The listing builds one solid part. Answer for the finished solid, in the listing's coordinates (mm). A direction names the side the tool comes from. Give positions to 0.01 mm unless a question says otherwise; leave off trailing zeros. Order: outer loops, then holes, each group sorted by start corner. A loop starts at its lowest first (then second) coordinate and runs counter-clockwise, first axis right, second up. Notation, with made-up numbers: (37, 85) - (77, 85) arc R25 ccw to (77, 109) - close; hole circle Ø6 at (-25.75, -34.75). An arc over 180 degrees is marked (long way). Answer as CSV lines item,"result". Start each with the question number.
1. Which of the six approach directions +Z, -Z, +X, -X, +Y, -Y give full straight-line access (tool end or side, diameter ignored) to faces 1 (the cylindrical face through (-1.729, -1.502, -4.396)), 2 (the flat face through (0, -4.5, 0)), 3 (the flat face through (-2, -1.2, -3))?
2. Section A-A on z = -7 is taken. Give the vertices of the cut face in (x, y) (3 decimals).
3. Flat-ended cylindrical pins translate along their axes: pin 1 (5 mm diameter, centred on y = -0.5, z = -6, fed in from -X) (3 decimals); pin 2 (1.7 mm diameter, centred on x = 1.75, y = 0, fed in from +Z); pin 3 (2 mm diameter, centred on x = -2, z = -5, fed in from +Y). Find the tip coordinate at first contact, or state that the pin passes through.
4. Consider line 1 along Y through (x, z) = (0.5, 0.5); line 2 along X through (y, z) = (-0.5, -3.75) (3 decimals); line 3 along Y through (x, z) = (-1.75, -7.2). Determine where each line is inside the solid, lowest interval first. Write a range as [from, to].
5. Section C-C on z = -2.25 is taken. Give the vertices of the cut face in (x, y) (3 decimals).
6. Section D-D on y = 0 is taken. Count the separate pieces of the cut face and the enclosed holes in it, and give its area (3 significant figures).
7. Determine the mould class of faces 4 (the flat face through (1.8, 1.3, -7.65)), 5 (the flat face through (-2.65, 0, -2)), 6 (the flat face through (3.5, -0.1, -0.7)) for opening direction X: +X half, -X half, draft (parallel to the pull), parting line (faces both ways), or undercut.
from build123d import *

# Parameters (mm, degrees)
SKETCH_1_W                     = 3.125
SKETCH_1_H                     = 10.4
EXTRUDE_1_DEPTH                = 2.1
CUT_EXTRUDE_1_REACH            = 8.249
SKETCH_2_W                     = 6.25
SKETCH_2_H                     = 9
SKETCH_3_W                     = 1.55
SKETCH_3_H                     = 0.7
CUT_EXTRUDE_2_DEPTH            = 1.05
SKETCH_5_W                     = 1.55
SKETCH_5_H                     = 0.7
CUT_EXTRUDE_4_DEPTH            = 1.05
EXTRUDE_3_DEPTH                = 6.6
SKETCH_9_W                     = 2.8
SKETCH_9_H                     = 7.7
EXTRUDE_4_DEPTH                = 1.3
CUT_EXTRUDE_6_REACH            = 11.424
SKETCH_11_W                    = 1.8
SKETCH_11_H                    = 6.7
CUT_EXTRUDE_9_REACH            = 11.047
SKETCH_14_W                    = 1.8
SKETCH_14_H                    = 2.4
CUT_EXTRUDE_11_REACH           = 14.749
SKETCH_16_W                    = 1.55
SKETCH_16_H                    = 0.6
CUT_EXTRUDE_12_REACH           = 14.749
SKETCH_17_W                    = 1.55
SKETCH_17_H                    = 0.6
EXTRUDE_6_DEPTH                = 0.375
SKETCH_21_W                    = 0.8
SKETCH_21_H                    = 2.5
EXTRUDE_8_DEPTH                = 1.3
HOLE_WIZARD_2_1_2_1_2_D        = 2.1
HOLE_WIZARD_2_1_2_1_2_DEPTH    = 1.2
HOLE_WIZARD_1_5_1_5_1_D        = 1.5
HOLE_WIZARD_1_5_1_5_1_DEPTH    = 2.000025
FILLET_1_R                     = 0.3
PATTERN_LINEAR_1_COUNT         = 2
PATTERN_LINEAR_1_PITCH         = 3.5
FILLET_1_OF_PATTERN_LINEAR_1_R = 0.3


with BuildPart() as part:
    # Эскиз1 → Бобышка-Вытянуть1 (new body)
    with BuildSketch(Plane.XY.offset(1.05)):
        with Locations((-1.5625, 0)):
            Rectangle(SKETCH_1_W, SKETCH_1_H)
    extrude_1 = extrude(amount=-EXTRUDE_1_DEPTH)

    # Эскиз2 → Вырез-Вытянуть1 (cut, up to next)
    with BuildSketch(Plane(origin=(0, 0, -0.45), x_dir=(-1, 0, 0), z_dir=(0, 0, -1)), mode=Mode.PRIVATE) as cut_extrude_1_sk1:
        Rectangle(SKETCH_2_W, SKETCH_2_H)
    cut_extrude_1_tool1 = extrude(cut_extrude_1_sk1.sketch, amount=-CUT_EXTRUDE_1_REACH, mode=Mode.PRIVATE) & part.part
    cut_extrude_1 = cut_extrude_1_tool1.solids().sort_by_distance((0, 0, -0.45))[0]
    add(cut_extrude_1, mode=Mode.SUBTRACT)

    # Эскиз3 → Вырез-Вытянуть2 (cut)
    with BuildSketch(Plane(origin=(0, 0, -0.45), x_dir=(-1, 0, 0), z_dir=(0, 0, -1))):
        with Locations((1.75, 4.85)):
            Rectangle(SKETCH_3_W, SKETCH_3_H)
    cut_extrude_2 = extrude(amount=-CUT_EXTRUDE_2_DEPTH, mode=Mode.SUBTRACT)

    # Эскиз5 → Вырез-Вытянуть4 (cut)
    with BuildSketch(Plane(origin=(0, 0, -0.45), x_dir=(-1, 0, 0), z_dir=(0, 0, -1))):
        with Locations((1.75, -4.85)):
            Rectangle(SKETCH_5_W, SKETCH_5_H)
    cut_extrude_4 = extrude(amount=-CUT_EXTRUDE_4_DEPTH, mode=Mode.SUBTRACT)

    # Эскиз8 → Бобышка-Вытянуть3 (add)
    with BuildSketch(Plane(origin=(0, 0, -7.65), x_dir=(-1, 0, 0), z_dir=(0, 0, -1))):
        with BuildLine():
            Line((3.125, 2.05), (0.375, 2.05))
            Line((0.375, 2.05), (0.375, -2.05))
            ThreePointArc((0.375, -2.05), (1.75, -1.502368755), (3.125, -2.05))
            Line((3.125, -2.05), (3.125, 2.05))
        make_face()
    extrude_3 = extrude(amount=-EXTRUDE_3_DEPTH)

    # Эскиз9 → Бобышка-Вытянуть4 (add)
    with BuildSketch(Plane.XY.offset(0.85)):
        with Locations((-1.75, 0)):
            Rectangle(SKETCH_9_W, SKETCH_9_H)
    extrude_4 = extrude(amount=-EXTRUDE_4_DEPTH)

    # Эскиз11 → Вырез-Вытянуть6 (cut, up to next)
    with BuildSketch(Plane(origin=(0, 0, -0.45), x_dir=(-1, 0, 0), z_dir=(0, 0, -1)), mode=Mode.PRIVATE) as cut_extrude_6_sk1:
        with Locations((1.75, 0)):
            Rectangle(SKETCH_11_W, SKETCH_11_H)
    cut_extrude_6_tool1 = extrude(cut_extrude_6_sk1.sketch, amount=-CUT_EXTRUDE_6_REACH, mode=Mode.PRIVATE) & part.part
    cut_extrude_6 = cut_extrude_6_tool1.solids().sort_by_distance((-1.75, 0, -0.45))[0]
    add(cut_extrude_6, mode=Mode.SUBTRACT)

    # Эскиз14 → Вырез-Вытянуть9 (cut, up to next)
    with BuildSketch(Plane(origin=(0, 0, -5.65), x_dir=(-1, 0, 0), z_dir=(0, 0, -1)), mode=Mode.PRIVATE) as cut_extrude_9_sk1:
        with Locations((1.75, 0)):
            Rectangle(SKETCH_14_W, SKETCH_14_H)
    cut_extrude_9_tool1 = extrude(cut_extrude_9_sk1.sketch, amount=-CUT_EXTRUDE_9_REACH, mode=Mode.PRIVATE) & part.part
    cut_extrude_9 = cut_extrude_9_tool1.solids().sort_by_distance((-1.75, 0, -5.65))[0]
    add(cut_extrude_9, mode=Mode.SUBTRACT)

    # Эскиз16 → Вырез-Вытянуть11 (cut, up to next)
    with BuildSketch(Plane(origin=(0, -4.5, 0), x_dir=(1, 0, 0), z_dir=(0, 1, 0)), mode=Mode.PRIVATE) as cut_extrude_11_sk1:
        with Locations((-1.75, 0.75)):
            Rectangle(SKETCH_16_W, SKETCH_16_H)
    cut_extrude_11_tool1 = extrude(cut_extrude_11_sk1.sketch, amount=-CUT_EXTRUDE_11_REACH, mode=Mode.PRIVATE) & part.part
    cut_extrude_11 = cut_extrude_11_tool1.solids().sort_by_distance((-1.75, -4.5, -0.75))[0]
    add(cut_extrude_11, mode=Mode.SUBTRACT)

    # Эскиз17 → Вырез-Вытянуть12 (cut, up to next)
    with BuildSketch(Plane.XZ.offset(-4.5), mode=Mode.PRIVATE) as cut_extrude_12_sk1:
        with Locations((-1.75, -0.75)):
            Rectangle(SKETCH_17_W, SKETCH_17_H)
    cut_extrude_12_tool1 = extrude(cut_extrude_12_sk1.sketch, amount=-CUT_EXTRUDE_12_REACH, mode=Mode.PRIVATE) & part.part
    cut_extrude_12 = cut_extrude_12_tool1.solids().sort_by_distance((-1.75, 4.5, -0.75))[0]
    add(cut_extrude_12, mode=Mode.SUBTRACT)

    # Эскиз19 → Бобышка-Вытянуть6 (add)
    with BuildSketch(Plane(origin=(-3.5, 0, 0), x_dir=(0, -1, 0), z_dir=(-1, 0, 0))):
        Polygon((1.65, -1.046361901), (5.2, -1.046361901), (5.2, 1.05), (4.5, 1.05), (4.5, -0.45), (-4.5, -0.45), (-4.5, 1.05), (-5.2, 1.05), (-5.2, -1.046361901), align=None)
    extrude_6 = extrude(amount=-EXTRUDE_6_DEPTH)

    # Эскиз21 → Бобышка-Вытянуть8 (add)
    with BuildSketch(Plane(origin=(0, 3.35, 0), x_dir=(1, 0, 0), z_dir=(0, 1, 0))):
        with Locations((-1.75, 6.4)):
            Rectangle(SKETCH_21_W, SKETCH_21_H)
    extrude_8 = extrude(amount=-EXTRUDE_8_DEPTH)

    # Диаметр отверстия Ø2.1 (2.1)2
    with Locations(Plane(origin=(0, 0, -7.65), x_dir=(-1, 0, 0), z_dir=(0, 0, -1))):
        with Locations((1.75, 0)):
            hole_wizard_2_1_2_1_2 = Hole(HOLE_WIZARD_2_1_2_1_2_D / 2, depth=HOLE_WIZARD_2_1_2_1_2_DEPTH)

    # Диаметр отверстия Ø1.5 (1.5)1
    with Locations(Plane.XY.offset(-5.65)):
        with Locations((-1.75, 0)):
            hole_wizard_1_5_1_5_1 = Hole(HOLE_WIZARD_1_5_1_5_1_D / 2, depth=HOLE_WIZARD_1_5_1_5_1_DEPTH)

    # Скругление1
    fillet_1_edges = [part.edges().sort_by_distance(p)[0] for p in [
        (-2.8, 0, -6.45),
    ]]
    fillet(fillet_1_edges, radius=FILLET_1_R - 0.0001)  # a hair under: the kernel refuses the full size

    # Линейный массив1: Бобышка-Вытянуть1, Вырез-Вытянуть1, Вырез-Вытянуть2, Вырез-Вытянуть4, Бобышка-Вытянуть3, Бобышка-Вытянуть4, Вырез-Вытянуть6, Вырез-Вытянуть9, Вырез-Вытянуть11, Вырез-Вытянуть12, Бобышка-Вытянуть6, Бобышка-Вытянуть8, Диаметр отверстия Ø2.1 (2.1)2, Диаметр отверстия Ø1.5 (1.5)1 ×2
    with Locations(*[(i * PATTERN_LINEAR_1_PITCH, 0, 0) for i in range(1, PATTERN_LINEAR_1_COUNT)]):
        add(extrude_1)
        add(cut_extrude_1, mode=Mode.SUBTRACT)
        add(cut_extrude_2, mode=Mode.SUBTRACT)
        add(cut_extrude_4, mode=Mode.SUBTRACT)
        add(extrude_3)
        add(extrude_4)
        add(cut_extrude_6, mode=Mode.SUBTRACT)
        add(cut_extrude_9, mode=Mode.SUBTRACT)
        add(cut_extrude_11, mode=Mode.SUBTRACT)
        add(cut_extrude_12, mode=Mode.SUBTRACT)
        add(extrude_6)
        add(extrude_8)
        add(hole_wizard_2_1_2_1_2, mode=Mode.SUBTRACT)
        add(hole_wizard_1_5_1_5_1, mode=Mode.SUBTRACT)

    # Скругление1 of Линейный массив1
    fillet_1_of_pattern_linear_1_edges = [part.edges().sort_by_distance(p)[0] for p in [
        (0.7, 0, -6.45),
    ]]
    fillet(fillet_1_of_pattern_linear_1_edges, radius=FILLET_1_OF_PATTERN_LINEAR_1_R - 0.0001)  # a hair under: the kernel refuses the full size


solid = part.part
Checks:
1,face 1,"-Z, -Y"
1,face 2,"+Z, +X, -X"
1,face 3,"+Z"
2,outline,"(-3.125, -2.05) arc R2 cw to (-0.375, -2.05) - (-0.375, 2.05) - (-1.35, 2.05) - (-1.35, 3.35) - (-2.15, 3.35) - (-2.15, 2.05) - (-3.125, 2.05) - close; (0.375, -2.05) arc R2 cw to (3.125, -2.05) - (3.125, 2.05) - (2.15, 2.05) - (2.15, 3.35) - (1.35, 3.35) - (1.35, 2.05) - (0.375, 2.05) - close; hole circle Ø2.1 at (-1.75, 0); hole circle Ø2.1 at (1.75, 0)"
3,pin 1,"stops at x = -3.125"
3,pin 2,"stops at z = -5.65"
3,pin 3,"stops at y = 3.35"
4,line 1,"y = [-5.2, -4.5], [-3.85, 3.85], [4.5, 5.2]"
4,line 2,"x = [-3.125, -2.65], [-0.85, -0.375], [0.375, 0.85], [2.65, 3.125]"
4,line 3,"y = [-1.5, -1.05], [1.05, 3.35]"
5,outline,"(-3.125, -2.05) arc R2 cw to (-0.375, -2.05) - (-0.375, 2.05) - (-3.125, 2.05) - close; (0.375, -2.05) arc R2 cw to (3.125, -2.05) - (3.125, 2.05) - (0.375, 2.05) - close; hole (-2.65, -1.2) - (-0.85, -1.2) - (-0.85, 1.2) - (-2.65, 1.2) - close; hole (0.85, -1.2) - (2.65, -1.2) - (2.65, 1.2) - (0.85, 1.2) - close"
6,separate pieces,"3"
6,enclosed holes,"0"
6,area,"17.0 mm²"
7,face 4,"draft"
7,face 5,"undercut"
7,face 6,"+X half"
